Geometry: final body of the model. Coordinates: model frame, mm. A direction names the side the tool comes from. Coordinates: 2 decimals unless noted, no trailing zeros. Loops run counter-clockwise (first coordinate to the right, second up) from the corner with the lowest first, then second, coordinate; pieces in that order, holes last. Notation, with made-up numbers: (27, 73.25) - (84, 73.25) arc R19 ccw to (84, 93.25) - close; hole circle Ø4 at (87.25, -30). An arc over 180 degrees is marked (long way). Put each result on its own line as item: value. Start each with the question number.
1) Draft query along Z for faces 5 (the cylindrical face through (26.455, 3.254, 9.246)), 6 (the flat face through (23.7, 1.638, 6.3)), 7 (the cylindrical face through (30.59, 3.3, 11.17)). Return one class per face: +Z half, -Z half, draft (parallel to the pull), parting line (faces both ways), or undercut.
2) Section C-C on y = 0. Output: boundary loops of the cut face in (x, z).
3) Contact query for flat-ended pins moving along their axis: pin 1 Ø5 at (x, y) = (18, 1) entering from -Z; pin 2 Ø2 at (x, z) = (23.5, 11) entering from +Y; pin 3 Ø3.5 at (x, y) = (-10.5, -3) entering from -Z; pin 4 Ø2 at (x, y) = (-5.13, 0) entering from +Z. Output: stop coordinate, or through.
4) Section B-B on z = 8.5. Output: boundary loops of the cut face in (x, y) (3 decimals), and give its area (3 significant figures).
5) Reachability of faces 1 (the flat face through (-9, 0, 6.35)), 2 (the flat face through (23.7, -4.915, 6.3)), 3 (the flat face through (24, 4.915, 5)), 4 (the flat face through (20.575, 0, 6)) from +Z, -Z, +X, -X, +Y, -Y: full face, straight path, thin tool, end or side. Return the list, or none.
6) Section D-D on z = 3. Output: boundary loops of the cut face in (x, y) (3 decimals), and give its area (3 significant figures).
7) Section A-A on x = 23. Output: boundary loops of the cut face in (y, z).
8) Material intervals for line 1 along X through (y, z) = (0, 7.5); line 2 along Y through (x, z) = (22, 10.75); line 3 along Y through (x, z) = (-4, 9.25) (3 decimals), sorted ascending. Write a range as from..to.
```python
from build123d import *

# Parameters (mm, degrees)
F0_R     = 3.81
F1_DEPTH = 12.7
F3_R     = 5.08
F2_R     = 2.921
F4_DEPTH = 16.9809
F6_DEPTH = 24.131
F7_R     = 1.6383
F8_DEPTH = 25.4


with BuildPart() as f1:
    # F0 (on Top) → F1 (new body)
    with BuildSketch(Plane.XY):
        with BuildLine():
            Line((11.376741, 12.065), (-12.94174, 12.065))
            Line((-12.94174, 12.065), (-12.94174, -12.065))
            Line((-12.94174, -12.065), (11.376741, -12.065))
            ThreePointArc((11.376741, -12.065), (17.201771, -10.067217), (20.574564, -4.9149))
            Line((20.574564, -4.9149), (32.037482, -4.9149))
            Line((32.037482, -4.9149), (32.037482, -1.6383))
            Line((32.037482, -1.6383), (20.574564, -1.6383))
            Line((20.574564, -1.6383), (20.574564, 1.6383))
            Line((20.574564, 1.6383), (32.037482, 1.6383))
            Line((32.037482, 1.6383), (32.037482, 4.9149))
            Line((32.037482, 4.9149), (20.574564, 4.9149))
            ThreePointArc((20.574564, 4.9149), (17.201771, 10.067217), (11.376741, 12.065))
        make_face()
        with Locations((8.26726, 0)):
            Circle(F0_R, mode=Mode.SUBTRACT)
    extrude(amount=F1_DEPTH)

    # F3
    f3_edges = [f1.edges().sort_by_distance(p)[0] for p in [
        (32.037482, -3.2766, 12.7),
        (32.037482, 3.2766, 12.7),
        (32.037482, -3.2766, 0),
        (32.037482, 3.2766, 0),
    ]]
    fillet(f3_edges, radius=F3_R)

    # F2 (on face) → F4 (cut, through all)
    with BuildSketch(Plane.XZ.offset(4.9149)):
        with Locations((26.8351, 6.35)):
            Circle(F2_R)
    extrude(amount=-F4_DEPTH, mode=Mode.SUBTRACT)

    # F5 (on face) → F6 (cut, through all)
    with BuildSketch(Plane.XZ.offset(12.065)):
        Polygon((-5.969032, 6.35), (-12.94174, 6.35), (-12.94174, 0), (11.376741, 0), (11.376741, 2.202417), align=None)
        Polygon((20.58756, 0), (11.376741, 2.202417), (11.376741, 0), align=None)
    extrude(amount=-F6_DEPTH, mode=Mode.SUBTRACT)

    # F7 (on face) → F8 (cut)
    with BuildSketch(Plane.XY.offset(12.7)):
        with Locations((-5.13124, 0)):
            Circle(F7_R)
    extrude(amount=-F8_DEPTH, mode=Mode.SUBTRACT)


solid = f1.part
```
Answer block:
1. face 5: undercut
1. face 6: draft
1. face 7: +Z half
2. outline: (-12.94, 6.35) - (-6.77, 6.35) - (-6.77, 12.7) - (-12.94, 12.7) - close; (-3.49, 5.76) - (4.46, 3.86) - (4.46, 12.7) - (-3.49, 12.7) - close; (12.08, 2.03) - (20.57, 0) - (20.57, 12.7) - (12.08, 12.7) - close
3. pin 1: stops at z = 0.02
3. pin 2: stops at y = 4.91
3. pin 3: stops at z = 6.35
3. pin 4: passes through
4. outline: (-12.942, -12.065) - (11.377, -12.065) arc R9.491 ccw to (20.575, -4.915) - (24.858, -4.915) - (24.858, -1.638) - (20.575, -1.638) - (20.575, 1.638) - (24.858, 1.638) - (24.858, 4.915) - (20.575, 4.915) arc R9.491 ccw to (11.377, 12.065) - (-12.942, 12.065) - close; (28.812, -4.915) - (31.961, -4.915) - (31.961, -1.638) - (28.812, -1.638) - close; (28.812, 1.638) - (31.961, 1.638) - (31.961, 4.915) - (28.812, 4.915) - close; hole circle Ø3.277 at (-5.131, 0); hole circle Ø7.62 at (8.267, 0)
4. area: 769 mm²
5. face 1: -Z, -X, +Y, -Y
5. face 2: +Z, -Z, +X, -Y
5. face 3: +Z, -Z, +X, +Y
5. face 4: +Z, -Z, +X
6. outline: (8.041, -12.065) - (11.377, -12.065) arc R9.491 ccw to (20.575, -4.915) - (31.592, -4.915) - (31.592, -1.638) - (20.575, -1.638) - (20.575, 1.638) - (31.592, 1.638) - (31.592, 4.915) - (20.575, 4.915) arc R9.491 ccw to (11.377, 12.065) - (8.041, 12.065) - (8.041, 3.803) arc R3.81 cw (long way) to (8.041, -3.803) - close
6. area: 316 mm²
7. outline: (-4.91, 0) - (-1.64, 0) - (-1.64, 12.7) - (-4.91, 12.7) - close; (1.64, 0) - (4.91, 0) - (4.91, 12.7) - (1.64, 12.7) - close
8. line 1: x = -12.94..-6.77, -3.49..4.46, 12.08..20.57
8. line 2: y = -4.91..-1.64, 1.64..4.91
8. line 3: y = -12.065..-1.185, 1.185..12.065
